Build history of the part. All positions in model axes, mm. A direction names the side the tool comes from. Round coordinates to 2 decimals unless told otherwise and drop trailing zeros. Write each loop counter-clockwise with the first axis right and the second up, starting at its lowest first coordinate (ties: lowest second). Pieces come first, ordered by that corner, then holes. Notation, with made-up numbers: (-25, -8.5) -> (3, -8.5) arc R20 cw to (3, -3.5) -> close; hole circle Ø6 at (-6, 32). An arc over 180 degrees is marked (long way). Answer as CSV lines item,"result".
from build123d import *

# Parameters (mm, degrees)
SKETCH_1_R          = 19.5
SKETCH_1_R_2        = 2
SKETCH_1_R_3        = 1.5
EXTRUDE_1_DEPTH     = 6.8
SKETCH_2_W          = 44
SKETCH_2_H          = 78
EXTRUDE_2_DEPTH     = 70
SKETCH_3_R          = 3
CUT_EXTRUDE_1_DEPTH = 12
CUT_EXTRUDE_2_DEPTH = 33
SKETCH_6_R          = 3
CUT_EXTRUDE_3_DEPTH = 12
CHAMFER_1_SIZE      = 2
FILLET_1_R          = 7
SKETCH_7_R          = 2
SKETCH_7_R_2        = 1.5
CUT_EXTRUDE_4_DEPTH = 22.8
SKETCH_8_R          = 3
CUT_EXTRUDE_5_DEPTH = 3.2


with BuildPart() as part:
    # 草图1 → 凸台-拉伸1 (new body)
    with BuildSketch(Plane(origin=(0, 0, 0), x_dir=(1, 0, 0), z_dir=(0, 1, 0))):
        Circle(SKETCH_1_R)
        with Locations((10.522208656, 6.075)):
            Circle(SKETCH_1_R_2, mode=Mode.SUBTRACT)
        with Locations((-10.522208656, 6.075)):
            Circle(SKETCH_1_R_2, mode=Mode.SUBTRACT)
        with Locations((0, -12.15)):
            Circle(SKETCH_1_R_2, mode=Mode.SUBTRACT)
        with Locations((0, 13.5)):
            Circle(SKETCH_1_R_3, mode=Mode.SUBTRACT)
        with Locations((11.691342951, -6.75)):
            Circle(SKETCH_1_R_3, mode=Mode.SUBTRACT)
        with Locations((-11.691342951, -6.75)):
            Circle(SKETCH_1_R_3, mode=Mode.SUBTRACT)
    extrude(amount=EXTRUDE_1_DEPTH)

    # 草图2 → 凸台-拉伸2 (add)
    with BuildSketch(Plane(origin=(0, 6.8, 0), x_dir=(1, 0, 0), z_dir=(0, 1, 0))):
        Rectangle(SKETCH_2_W, SKETCH_2_H)
    extrude(amount=EXTRUDE_2_DEPTH)

    # 草图3 → 切除-拉伸1 (cut)
    with BuildSketch(Plane(origin=(22, 0, 0), x_dir=(0, 0, -1), z_dir=(1, 0, 0))):
        with Locations((0, 14.8)):
            Circle(SKETCH_3_R)
        with Locations((-29.5, 14.8)):
            Circle(SKETCH_3_R)
        with Locations((29.5, 14.8)):
            Circle(SKETCH_3_R)
        Polygon((-39, 6.8), (-36.626907991, 21.8), (36.626907991, 21.8), (39, 6.8), (44.081826142, 6.8), (44.081826142, 83.498576474), (-44.081826142, 83.498576474), (-44.081826142, 6.8), align=None)
    extrude(amount=-CUT_EXTRUDE_1_DEPTH, mode=Mode.SUBTRACT)

    # 草图5 → 切除-拉伸2 (cut, through all)
    with BuildSketch(Plane(origin=(10, 0, 0), x_dir=(0, 0, -1), z_dir=(1, 0, 0))):
        Polygon((-39, 6.8), (-36.626907991, 21.8), (36.626907991, 21.8), (39, 6.8), (39, 76.8), (-39, 76.8), align=None)
    extrude(amount=-CUT_EXTRUDE_2_DEPTH, mode=Mode.SUBTRACT)

    # 草图6 → 切除-拉伸3 (cut)
    with BuildSketch(Plane.ZY.offset(22)):
        with Locations((-29.5, 14.8)):
            Circle(SKETCH_6_R)
        with Locations((0, 14.8)):
            Circle(SKETCH_6_R)
        with Locations((29.5, 14.8)):
            Circle(SKETCH_6_R)
    extrude(amount=-CUT_EXTRUDE_3_DEPTH, mode=Mode.SUBTRACT)

    # 倒角1
    chamfer_1_edges = [part.edges().sort_by_distance(p)[0] for p in [
        (-19.5, 6.8, 0),
    ]]
    chamfer(chamfer_1_edges, length=CHAMFER_1_SIZE)

    # 圆角1
    fillet_1_edges = [part.edges().sort_by_distance(p)[0] for p in [
        (0, 6.8, -39),
        (0, 6.8, 39),
    ]]
    fillet(fillet_1_edges, radius=FILLET_1_R)

    # 草图7 → 切除-拉伸4 (cut, through all)
    with BuildSketch(Plane(origin=(0, 21.8, 0), x_dir=(1, 0, 0), z_dir=(0, 1, 0))):
        with Locations((10.522208656, 6.075)):
            Circle(SKETCH_7_R)
        with Locations((11.691342951, -6.75)):
            Circle(SKETCH_7_R_2)
        with Locations((0, -12.15)):
            Circle(SKETCH_7_R)
        with Locations((-11.691342951, -6.75)):
            Circle(SKETCH_7_R_2)
        with Locations((-10.522208656, 6.075)):
            Circle(SKETCH_7_R)
        with Locations((0, 13.5)):
            Circle(SKETCH_7_R_2)
    extrude(amount=-CUT_EXTRUDE_4_DEPTH, mode=Mode.SUBTRACT)

    # 草图8 → 切除-拉伸5 (cut)
    with BuildSketch(Plane(origin=(0, 21.8, 0), x_dir=(1, 0, 0), z_dir=(0, 1, 0))):
        with Locations((0, 13.5)):
            Circle(SKETCH_8_R)
        with Locations((11.691342951, -6.75)):
            Circle(SKETCH_8_R)
        with Locations((-11.691342951, -6.75)):
            Circle(SKETCH_8_R)
    extrude(amount=-CUT_EXTRUDE_5_DEPTH, mode=Mode.SUBTRACT)


solid = part.part
1. Cut at A-A, the plane z = 0. Write the cut outline in (x, y).
Results found:
outline,"(-22, 6.8) -> (-21.5, 6.8) -> (-19.5, 4.8) -> (-19.5, 0) -> (19.5, 0) -> (19.5, 4.8) -> (21.5, 6.8) -> (22, 6.8) -> (22, 11.8) -> (10, 11.8) -> (10, 17.8) -> (22, 17.8) -> (22, 21.8) -> (-22, 21.8) -> (-22, 17.8) -> (-10, 17.8) -> (-10, 11.8) -> (-22, 11.8) -> close"
2. Drop flat-ended pins along their axis: pin 1 Ø1 at (x, y) = (-15, 2.5) entering from +Z; pin 2 Ø3.5 at (y, z) = (14.8, 0) entering from +X; pin 3 Ø4 at (x, z) = (1, 23) entering from -Y. Give the stop position or say it passes through.
Results found:
pin 1,"stops at z = 13.04"
pin 2,"stops at x = 10"
pin 3,"stops at y = 6.32"
3. Cut at B-B, the plane x = 11.5. Count the separate pieces of the cut face and the enclosed holes in it, then the cut area to 3 significant figures.
Results found:
separate pieces,"3"
enclosed holes,"3"
area,"1,090 mm2"
4. Which spindle directions (+Z, -Z, +X, -X, +Y, -Y) get a long thin tool onto all of the face, cutting with end or side? Do faces 1 (the flat face through (10, 15, 30)), 2 (the flat face through (-10, 15, 0)), 3 (the cylindrical face through (-0.26, 11.053, 10.167)), 4 (the cylindrical face through (-10.08, 20.22, 4.22)). Say none if no direction does.
Results found:
face 1,"+X"
face 2,"-X"
face 3,"+Y, -Y"
face 4,"+Y"
5. Probe line 1 along X through (y, z) = (7.5, -6); line 2 along X through (y, z) = (8.75, 6.75); line 3 along Z through (x, y) = (-0.5, 9). List the from-to ranges inside material, lowest first.
Results found:
line 1,"x = -22 to -12.52, -8.52 to 8.52, 12.52 to 22"
line 2,"x = -22 to -13.19, -10.19 to 10.19, 13.19 to 22"
line 3,"z = -35.9 to -14.91, -12.09 to 10.21, 14.09 to 35.9"
6. Mould opens along Z. For faces 5 (the conical face through (18, 5, 8)), 6 (the flat face through (-10, 15, 29)), 7 (the flat face through (0, 0, 0)) say: +Z half, -Z half, draft (parallel to the pull), parting line (faces both ways), or undercut.
Results found:
face 5,"parting line"
face 6,"undercut"
face 7,"draft"
7. Cut at D-D, the plane z = -29.5. Write the cut outline in (x, y), then the cut area to 3 significant figures.
Results found:
outline,"(-22, 6.8) -> (22, 6.8) -> (22, 11.8) -> (10, 11.8) -> (10, 17.8) -> (22, 17.8) -> (22, 21.8) -> (-22, 21.8) -> (-22, 17.8) -> (-10, 17.8) -> (-10, 11.8) -> (-22, 11.8) -> close"
area,"516 mm2"
